For this review, take the finished solid that the model builds, in its own axes (mm). A direction names the side the tool comes from. Give positions to 0.01 mm unless a question says otherwise; leave off trailing zeros. Write each loop counter-clockwise with the first axis right and the second up, starting at its lowest first coordinate (ties: lowest second). Pieces come first, ordered by that corner, then holes.
1) We need section D-D on x = 12.7. Give the boundary of the cut face in (y, z), and give its area (3 significant figures).
2) Draft analysis for pull direction Z (two halves, no side actions). For faces 1 (the face through (26, 3, 0)), 2 (the face through (0, 3, -15)), 3 (the face through (19, 3, -48.934)), 4 (the face through (3.5, 3.13, -37.57)), state which applies: pulls with the +Z half, pulls with the -Z half, needs draft (parallel to the pull), parting line crosses it, or undercut.
3) We need section C-C on x = 31.75. Give the boundary of the cut face in (y, z).
4) Machinability: for faces 5 (the face through (39.142, 3.131, -40.475)), 6 (the face through (19, 3, -42.457)), which of the approach directions +Z, -Z, +X, -X, +Y, -Y give a long, thin tool a straight path to every point of the face, cutting with its end or side? Answer none if there is none.
5) We need section B-B on z = -12.7. Give the boundary of the cut face in (x, y).
6) We need section A-A on y = 3.75. Give the number of separate pieces and of enclosed holes in the cut face, and give its area (3 significant figures).
7) Wall thickness on line 1 along X through (y, z) = (2, -19.05); line 2 along X through (y, z) = (3, -12.7); line 3 along X through (y, z) = (4.25, -7.5): over which ranges is each line inside the solid? List them lowest first.
from build123d import *

# Parameters (mm, degrees)
SKETCH1_R           = 2.032
SKETCH1_W           = 6.477
SKETCH1_H           = 6.477
BOSS_EXTRUDE1_DEPTH = 6.35
FILLET1_R           = 6.35


with BuildPart() as part:
    # Sketch1 → Boss-Extrude1 (new body)
    with BuildSketch(Plane(origin=(0, 0, 0), x_dir=(1, 0, 0), z_dir=(0, 1, 0))):
        with BuildLine():
            Line((0, 25.4), (6.844498349, 49.204945244))
            ThreePointArc((6.844498349, 49.204945244), (16.662090732, 58.169055341), (29.096336444, 53.464810065))
            Line((29.096336444, 53.464810065), (50.8, 25.4))
            Line((50.8, 25.4), (50.8, 0))
            Line((50.8, 0), (0, 0))
            Line((0, 0), (0, 25.4))
        make_face()
        with Locations(Location((6.35, 6.35, 0), (0, 0, 270))):
            Circle(SKETCH1_R, mode=Mode.SUBTRACT)
        with Locations(Location((19.05, 6.35, 0), (0, 0, 270))):
            Circle(SKETCH1_R, mode=Mode.SUBTRACT)
        with Locations(Location((31.75, 6.35, 0), (0, 0, 270))):
            Circle(SKETCH1_R, mode=Mode.SUBTRACT)
        with Locations(Location((44.45, 6.35, 0), (0, 0, 270))):
            Circle(SKETCH1_R, mode=Mode.SUBTRACT)
        with Locations(Location((19.05, 19.05, 0), (0, 0, 270))):
            Circle(SKETCH1_R, mode=Mode.SUBTRACT)
        with Locations(Location((31.75, 19.05, 0), (0, 0, 270))):
            Circle(SKETCH1_R, mode=Mode.SUBTRACT)
        with Locations(Location((44.45, 19.05, 0), (0, 0, 270))):
            Circle(SKETCH1_R, mode=Mode.SUBTRACT)
        with Locations(Location((6.35, 19.05, 0), (0, 0, 270))):
            Circle(SKETCH1_R, mode=Mode.SUBTRACT)
        with Locations(Location((12.7, 12.7, 0), (0, 0, 270))):
            Circle(SKETCH1_R, mode=Mode.SUBTRACT)
        with Locations(Location((25.4, 12.7, 0), (0, 0, 270))):
            Circle(SKETCH1_R, mode=Mode.SUBTRACT)
        with Locations(Location((38.1, 12.7, 0), (0, 0, 270))):
            Circle(SKETCH1_R, mode=Mode.SUBTRACT)
        with Locations((19.05, 45.695567884)):
            Rectangle(SKETCH1_W, SKETCH1_H, mode=Mode.SUBTRACT)
    extrude(amount=BOSS_EXTRUDE1_DEPTH)

    # Fillet1
    fillet1_edges = [part.edges().sort_by_distance(p)[0] for p in [
        (0, 3.175, -25.4),
        (50.8, 3.175, -25.4),
        (50.8, 3.175, 0),
        (0, 3.175, 0),
    ]]
    fillet(fillet1_edges, radius=FILLET1_R)


solid = part.part
Results list:
1. outline: (0, -56.69) - (6.35, -56.69) - (6.35, -14.73) - (0, -14.73) - close; (0, -10.67) - (6.35, -10.67) - (6.35, 0) - (0, 0) - close
1. area: 334 mm2
2. face 1: pulls with the +Z half
2. face 2: needs draft
2. face 3: undercut
2. face 4: pulls with the -Z half
3. outline: (0, -50.03) - (6.35, -50.03) - (6.35, -21.08) - (0, -21.08) - close; (0, -17.02) - (6.35, -17.02) - (6.35, -8.38) - (0, -8.38) - close; (0, -4.32) - (6.35, -4.32) - (6.35, 0) - (0, 0) - close
4. face 5: -Z, +X, +Y, -Y
4. face 6: +Y, -Y
5. outline: (0, 0) - (10.67, 0) - (10.67, 6.35) - (0, 6.35) - close; (14.73, 0) - (23.37, 0) - (23.37, 6.35) - (14.73, 6.35) - close; (27.43, 0) - (36.07, 0) - (36.07, 6.35) - (27.43, 6.35) - close; (40.13, 0) - (50.8, 0) - (50.8, 6.35) - (40.13, 6.35) - close
6. separate pieces: 1
6. enclosed holes: 12
6. area: 2,160 mm2
7. line 1: x = 0 to 4.32, 8.38 to 17.02, 21.08 to 29.72, 33.78 to 42.42, 46.48 to 50.8
7. line 2: x = 0 to 10.67, 14.73 to 23.37, 27.43 to 36.07, 40.13 to 50.8
7. line 3: x = 0 to 4.67, 8.03 to 17.37, 20.73 to 30.07, 33.43 to 42.77, 46.13 to 50.8
